The model under review builds one solid part; all positions refer to its coordinate system, in mm. Face numbers are marked on the shaded views. A direction names the side the tool comes from. Give positions to 0.01 mm unless a question says otherwise; leave off trailing zeros. Loops run counter-clockwise (first coordinate to the right, second up) from the corner with the lowest first, then second, coordinate; pieces in that order, holes last. Notation, with made-up numbers: (70.25, -29) - (83.25, -29) arc R7 cw to (83.25, -19) - close; hole circle Ø9 at (60, 72). An arc over 180 degrees is marked (long way). Return JSON: item names as keys, results as strings. Group by question number.
```python
from build123d import *

# Parameters (mm, degrees)
SKETCH_R      = 2.5
EXTRUDE_DEPTH = 10


with BuildPart() as part:
    # Sketch → Extrude (new body)
    with BuildSketch(Plane.XY):
        with BuildLine():
            ThreePointArc((5, 0), (0, 5), (-5, 0))
            Line((-5, 0), (-5, -16.5))
            ThreePointArc((-5, -16.5), (0, -21.5), (5, -16.5))
            Line((5, 0), (5, -16.5))
        make_face()
        Circle(SKETCH_R, mode=Mode.SUBTRACT)
        with BuildLine():
            ThreePointArc((-2.399039, -16.432516), (0.266373, -19.199789), (3.000118, -16.5))
            Line((3.000118, -16.5), (3.000118, -12.179214))
            ThreePointArc((3.000118, -12.179214), (0.263808, -9.479458), (-2.398906, -12.251828))
            ThreePointArc((-2.399039, -16.432516), (-1.949453, -14.342186), (-2.398906, -12.251828))
        make_face(mode=Mode.SUBTRACT)
        with BuildLine():
            ThreePointArc((-3.51031, -17.45064), (-2.449453, -14.342024), (-3.51031, -11.233408))
            Line((-3.51031, -11.233408), (-3.51031, -17.45064))
        make_face(mode=Mode.SUBTRACT)
    extrude(amount=EXTRUDE_DEPTH)


solid = part.part
```
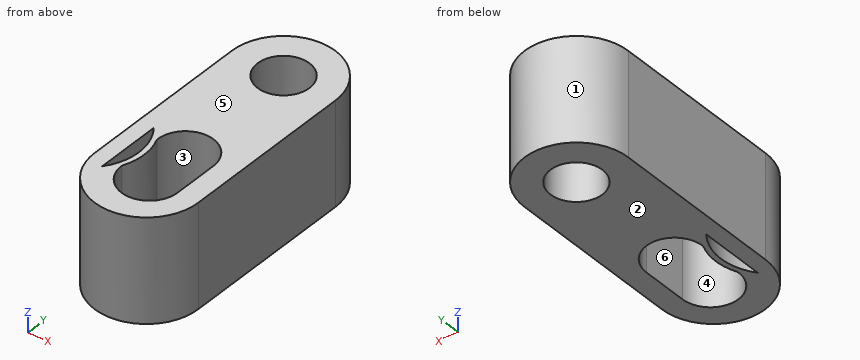
1) For pin 1 Ø2 at (x, z) = (2, 1.5) entering from +Y; pin 2 Ø2 at (x, z) = (-2.5, 2) entering from +Y, all flat-tipped, find the tip position at first contact; note any pin that passes through.
2) We need section C-C, the plane z = 8.5. Write out the cut boundary in (x, y) (3 decimals), plus the area to 3 significant figures.
3) We need section B-B, the plane x = -1. Write out the cut boundary in (y, z), plus the area to 3 significant figures.
4) To check wall thickness, follow line 1 (Y direction, x = 0, z = 7.5); line 2 (Y direction, x = -0.25, z = 2.25); line 3 (X direction, y = -18.75, z = 2). State the ranges of each line that lie inside material, in increasing order.
5) Tool access review of the marked faces 5 and 6: name each direction out of +Z, -Z, +X, -X, +Y, -Y from which nothing blocks a thin tool from reaching the whole face with its end or side.
6) We need section D-D, the plane y = -11.5. Write out the cut boundary in (x, z), plus the area to 3 significant figures.
7) We need section A-A, the plane y = 2. Write out the cut boundary in (x, z).
8) Draft analysis for pull direction X (two halves, no side actions). For the marked faces 1, 2, 3 and 4, state which applies: +X half, -X half, draft (parallel to the pull), parting line (faces both ways), or undercut.
Findings:
{
 "1": {"pin 1": "stops at y = 4.9", "pin 2": "stops at y = 4.77"},
 "2": {"outline": "(-5, -16.5) arc R5 ccw to (5, -16.5) - (5, 0) arc R5 ccw to (-5, 0) - close; hole (-3.51, -17.451) arc R5.085 ccw to (-3.51, -11.233) - close; hole circle Ø5 at (0, 0); hole (-2.399, -16.433) arc R2.7 ccw (long way) to (3, -16.5) - (3, -12.179) arc R2.7 ccw (long way) to (-2.399, -12.252) arc R5.085 cw to start", "area": "174 mm^2"},
 "3": {"outline": "(-21.4, 0) - (-18.87, 0) - (-18.87, 10) - (-21.4, 10) - close; (-9.81, 0) - (-2.29, 0) - (-2.29, 10) - (-9.81, 10) - close; (2.29, 0) - (4.9, 0) - (4.9, 10) - (2.29, 10) - close", "area": "127 mm^2"},
 "4": {"line 1": "y = -21.5 to -19.18, -9.5 to -2.5, 2.5 to 5", "line 2": "y = -21.49 to -19.14, -9.54 to -2.49, 2.49 to 4.99", "line 3": "x = -4.47 to -1.19, 1.79 to 4.47"},
 "5": {"face 5": "+Z, +X, -X, +Y, -Y", "face 6": "+Z, -Z"},
 "6": {"outline": "(-5, 0) - (-3.51, 0) - (-3.51, 10) - (-5, 10) - close; (-3.32, 0) - (-2.31, 0) - (-2.31, 10) - (-3.32, 10) - close; (2.91, 0) - (5, 0) - (5, 10) - (2.91, 10) - close", "area": "45.8 mm^2"},
 "7": {"outline": "(-4.58, 0) - (-1.5, 0) - (-1.5, 10) - (-4.58, 10) - close; (1.5, 0) - (4.58, 0) - (4.58, 10) - (1.5, 10) - close"},
 "8": {"face 1": "parting line", "face 2": "draft", "face 3": "undercut", "face 4": "undercut"}
}
